Check sheet for the modelled part. Datum: model origin and axes. Units: mm. A direction names the side the tool comes from. Round coordinates to 2 decimals unless told otherwise and drop trailing zeros. Order: outer loops, then holes, each group sorted by start corner. A loop starts at its lowest first (then second) coordinate and runs counter-clockwise, first axis right, second up. Notation, with made-up numbers: (32, 50) -> (82, 50) arc R9 cw to (82, 64) -> close; hole circle Ø1 at (8, 13). An arc over 180 degrees is marked (long way). Answer in a Markdown table with one row per item. Add a question column.
1. Sectioned sample at B-B, the plane z = -48. Record the boundary of the cut face in (x, y).
2. Draft check along Z on faces 3 (the flat face through (-49, 0, 1)), 4 (the cylindrical face through (-101.507, 1.975, -17.391)), 5 (the flat face through (-102, 0, -29)). Enter one of: +Z half, -Z half, draft (parallel to the pull), parting line (faces both ways), or undercut.
3. Access from +Z, -Z, +X, -X, +Y, -Y to the whole of each face (thin tool, end or side, straight path). Record for faces 1 (the flat face through (-101, 0, -30)), 2 (the cylindrical face through (5, -0.1, 0.5)).
4. Material ranges on L1, parallel to X at y = 0, z = 0.7; L2, parallel to Z at x = -60.5, y = -1; L3, parallel to X at y = -1.25, z = -4.5, recorded low to high. Write a range as from..to.
5. Depth check by flat-ended pin: P1, Ø3, axis at x = -45.5, y = -0.5, coming from the -Z side; P2, Ø1, axis at y = 2.5, z = -57.5, coming from the +X side; P3, Ø4, axis at y = -1.5, z = -56.5, coming from the -X side; P4, Ø5, axis at y = 3, z = -63, coming from the +X side. Enter the tip coordinate at first touch or a pass-through.
6. Sectioned sample at A-A, the plane x = -5. Record the boundary of the cut face in (y, z).
```python
from build123d import *

# Parameters (mm, degrees)
BOSS_EXTRUDE1_DEPTH     = 5
SKETCH2_R               = 5
SKETCH2_R_2             = 3.088913235
BOSS_EXTRUDE2_DEPTH     = 1
SKETCH3_R               = 3.088913235
CUT_EXTRUDE1_DEPTH      = 1
CUT_EXTRUDE2_DEPTH      = 1
CUT_EXTRUDE2_DEPTH_BACK = 10


with BuildPart() as part:
    # Sketch1 → Boss-Extrude1 (new body, symmetric)
    with BuildSketch(Plane(origin=(0, 0, 0), x_dir=(1, 0, 0), z_dir=(0, 1, 0))):
        Polygon((0, 0), (-101, 0), (-101, 84.981911775), (-102, 84.981911775), (-102, -1), (0, -1), align=None)
    extrude(amount=BOSS_EXTRUDE1_DEPTH, both=True)

    # Sketch2 → Boss-Extrude2 (add)
    with BuildSketch(Plane.XY.offset(1)):
        Circle(SKETCH2_R)
        Circle(SKETCH2_R_2, mode=Mode.SUBTRACT)
    extrude(amount=-BOSS_EXTRUDE2_DEPTH)

    # Sketch3 → Cut-Extrude1 (cut)
    with BuildSketch(Plane.XY.offset(1)):
        Circle(SKETCH3_R)
    extrude(amount=-CUT_EXTRUDE1_DEPTH, mode=Mode.SUBTRACT)

    # Sketch4 → Cut-Extrude2 (cut, two sides)
    with BuildSketch(Plane.ZY.offset(102)) as cut_extrude2_sk:
        with BuildLine():
            Line((-84.981911775, 5), (-84.981911775, 1))
            Line((-84.981911775, 1), (-34.527427825, 1))
            ThreePointArc((-34.527427825, 1), (-17.14825011, 2.003332972), (0, 5))
            Line((0, 5), (-84.981911775, 5))
        make_face()
        with BuildLine():
            Line((-34.527427825, -1), (-84.981911775, -1))
            Line((-84.981911775, -1), (-84.981911775, -5))
            Line((-84.981911775, -5), (0, -5))
            ThreePointArc((0, -5), (-17.14825011, -2.003332972), (-34.527427825, -1))
        make_face()
    extrude(amount=CUT_EXTRUDE2_DEPTH, mode=Mode.SUBTRACT)
    extrude(cut_extrude2_sk.sketch, amount=-CUT_EXTRUDE2_DEPTH_BACK, mode=Mode.SUBTRACT)


solid = part.part
```
Answer key:
| question | item | result |
|---|---|---|
| 1 | outline | (-102, -1) -> (-101, -1) -> (-101, 1) -> (-102, 1) -> close |
| 2 | face 3 | +Z half |
| 2 | face 4 | -Z half |
| 2 | face 5 | draft |
| 3 | face 1 | -Z, +X, +Y, -Y |
| 3 | face 2 | +Z, -Z, +X |
| 4 | L1 | x = -102..-3.09, 3.09..5 |
| 4 | L2 | z = 0..1 |
| 4 | L3 | x = -102..-101 |
| 5 | P1 | stops at z = 0 |
| 5 | P2 | passes through |
| 5 | P3 | stops at x = -102 |
| 5 | P4 | stops at x = -101 |
| 6 | outline | (-5, 0) -> (5, 0) -> (5, 1) -> (-5, 1) -> close |
